Design review of the part shown in the three views and the two pictorial views. Dimensions are in mm from the part's minimum x, y and z. Round coordinates to 2 decimals unless told otherwise and drop trailing zeros. Order: outer loops, then holes, each group sorted by start corner. A loop starts at its lowest first (then second) coordinate and runs counter-clockwise, first axis right, second up. Notation, with made-up numbers: (-15.75, 43.5) - (-8.75, 43.5) arc R36 ccw to (-8.75, 80.5) - close; hole circle Ø10 at (-28, 9). An arc over 180 degrees is marked (long way). Use CSV: the item, a comma, the result in double quotes.
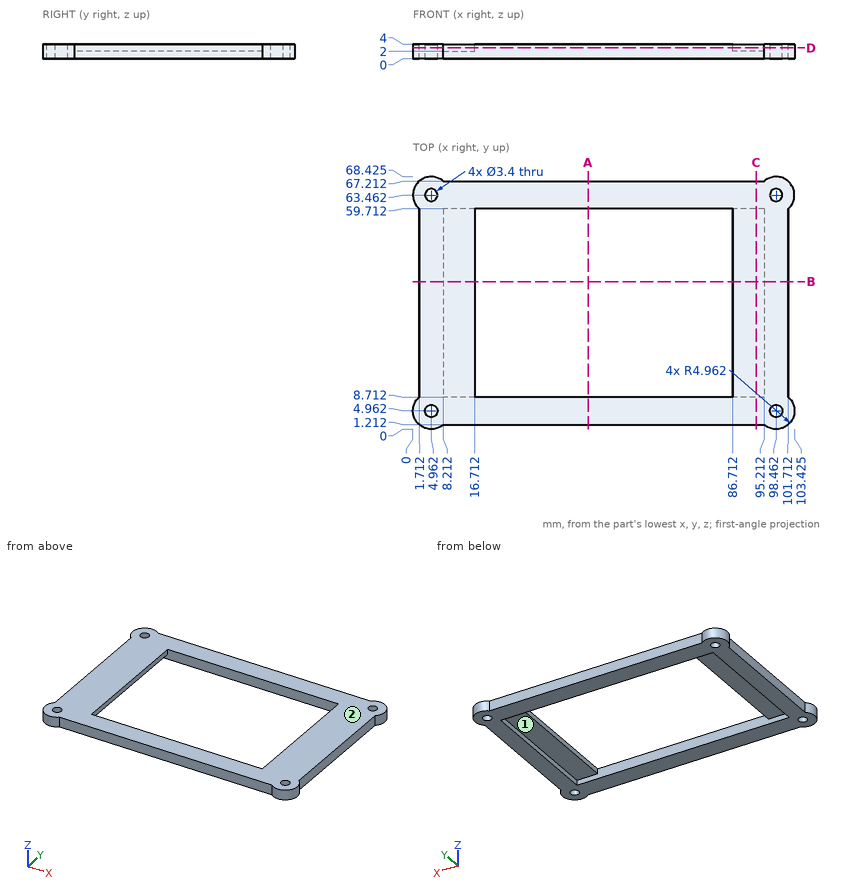
1) We need section D-D (z = 2.95). Give the boundary of the cut face in (x, y) (1 decimal).
Data:
outline,"(1.7, 8.7) arc R5 ccw to (8.2, 1.2) - (95.2, 1.2) arc R5 ccw to (101.7, 8.7) - (101.7, 59.7) arc R5 ccw to (95.2, 67.2) - (8.2, 67.2) arc R5 ccw to (1.7, 59.7) - close; hole circle Ø3.4 at (5, 5); hole circle Ø3.4 at (5, 63.5); hole (16.7, 8.7) - (86.7, 8.7) - (86.7, 59.7) - (16.7, 59.7) - close; hole circle Ø3.4 at (98.5, 5); hole circle Ø3.4 at (98.5, 63.5)"
2) To check wall thickness, follow L1, parallel to Y at x = 98.5, z = 3.1 (1 decimal); L2, parallel to X at y = 53, z = 3.45; L3, parallel to Y at x = 32, z = 2.3. State the ranges of each line that lie inside material, in increasing order. Write a range as from..to.
Data:
L1,"y = 0..3.3, 6.7..61.8, 65.2..68.4"
L2,"x = 1.71..16.71, 86.71..101.71"
L3,"y = 1.21..8.71, 59.71..67.21"
3) We need section B-B (y = 40). Give the boundary of the cut face in (x, z).
Data:
outline,"(1.71, 0) - (8.21, 0) - (8.21, 2) - (16.71, 2) - (16.71, 4) - (1.71, 4) - close; (86.71, 2) - (95.21, 2) - (95.21, 0) - (101.71, 0) - (101.71, 4) - (86.71, 4) - close"
4) The part is to be moulded in two halves that separate along X. For the marked faces 1 and 2, say which applies: +X half, -X half, draft (parallel to the pull), parting line (faces both ways), or undercut.
Data:
face 1,"undercut"
face 2,"draft"
5) Insertion check: pin 1 Ø10 at (x, y) = (19, 56.5) entering from -Z; pin 2 Ø1.2 at (x, z) = (49.5, 2.5) entering from +Y; pin 3 Ø3 at (x, y) = (98.46, 4.96) entering from -Z; pin 4 Ø1 at (y, z) = (25, 0.5) entering from +X. Each pin has a flat end and moves straight along its axis. Give the tip position at first contact, or say it passes through.
Data:
pin 1,"stops at z = 0"
pin 2,"stops at y = 67.21"
pin 3,"passes through"
pin 4,"stops at x = 101.71"
6) We need section A-A (x = 47.5). Give the boundary of the cut face in (y, z), then the cut area to 3 significant figures.
Data:
outline,"(1.21, 0) - (8.71, 0) - (8.71, 4) - (1.21, 4) - close; (59.71, 0) - (67.21, 0) - (67.21, 4) - (59.71, 4) - close"
area,"60.0 mm2"
7) We need section C-C (x = 93). Give the boundary of the cut face in (y, z).
Data:
outline,"(1.21, 0) - (8.71, 0) - (8.71, 2) - (59.71, 2) - (59.71, 0) - (67.21, 0) - (67.21, 4) - (1.21, 4) - close"
